from build123d import *

# Parameters (mm, degrees)
SKETCH2_R          = 1.5875
CUT_EXTRUDE1_DEPTH = 13.7


with BuildPart() as part:
    # Sketch1 → Revolve1 (revolve)
    with BuildSketch(Plane.XY):
        Polygon((-6.35, 0), (-6.35, 5.475), (-4.05, 3.175), (-2, 3.175), (-2, 2.675), (2, 2.675), (2, 3.175), (4.05, 3.175), (6.35, 5.475), (6.35, 0), align=None)
    revolve(axis=Axis((-93.951812963, 0, 0), (1, 0, 0)))

    # Sketch2 → Cut-Extrude1 (cut, through all)
    with BuildSketch(Plane.ZY.offset(6.35)):
        Circle(SKETCH2_R)
    extrude(amount=-CUT_EXTRUDE1_DEPTH, mode=Mode.SUBTRACT)


solid = part.part
The listing builds one solid part. Answer for the finished solid, in the listing's coordinates (mm). A direction names the side the tool comes from. Coordinates: 2 decimals unless noted, no trailing zeros. Answer in a Markdown table with one row per item. Add a question column.
Item 1: Find the intervals of material crossed by L1, parallel to X at y = -0.5, z = -3; L2, parallel to Y at x = -2.25, z = 1.25; L3, parallel to Y at x = 3.25, z = -2.75, in increasing order. Write a range as from..to.
Item 2: Determine the mould class of faces 3 (the face through (0.03, -0.58, -2.61)), 4 (the face through (-0.09, -1.55, -0.34)), 5 (the face through (-2, -2, -2)) for opening direction Y: +Y half, -Y half, draft (parallel to the pull), parting line (faces both ways), or undercut.
Item 3: Each of these flat-tipped pins is pushed along its axis until it touches: P1, Ø1.5, axis at x = -3, z = 1, coming from the +Y side; P2, Ø5, axis at x = 2.5, z = 1, coming from the +Y side; P3, Ø2, axis at x = -2, y = -3, coming from the -Z side; P4, Ø3, axis at y = 0, z = 0, coming from the -X side. Where does it stop, or does it pass through?
Item 4: Which of the six approach directions +Z, -Z, +X, -X, +Y, -Y give full straight-line access (tool end or side, diameter ignored) to faces 1 (the face through (6.35, -1.3, 1.3)), 2 (the face through (2, 2, -2))?
Result set:
| question | item | result |
|---|---|---|
| 1 | L1 | x = -6.35..-2, 2..6.35 |
| 1 | L2 | y = -2.92..-0.98, 0.98..2.92 |
| 1 | L3 | y = -1.59..1.59 |
| 2 | face 3 | parting line |
| 2 | face 4 | undercut |
| 2 | face 5 | draft |
| 3 | P1 | stops at y = 3.17 |
| 3 | P2 | stops at y = 4.05 |
| 3 | P3 | stops at z = -2.47 |
| 3 | P4 | passes through |
| 4 | face 1 | +Z, -Z, +X, +Y, -Y |
| 4 | face 2 | none |
